Build history of the part. All positions in model axes, mm. A direction names the side the tool comes from. Give positions to 0.01 mm unless a question says otherwise; leave off trailing zeros. Loops run counter-clockwise (first coordinate to the right, second up) from the corner with the lowest first, then second, coordinate; pieces in that order, holes last. Notation, with made-up numbers: (-37, -31.5) -> (4, -31.5) arc R9 ccw to (4, -21.5) -> close; hole circle Ø5 at (68.5, 64.25). An arc over 180 degrees is marked (long way). Answer as a JSON object with one key per item and string values. Group by question number.
Q1. Wall check: probe 1 along X at (y, z) = (-13, 24.5); probe 2 along Y at (x, z) = (7.5, 29.5); probe 3 along Y at (x, z) = (-7, 32). Give the ranges that are in metal, low to high. Write a range as from..to.
Q2. Band-saw the part on B-B, the plane z = 5. Write the cut outline in (x, y), plus the area to 3 significant figures.
Q3. Band-saw the part on D-D, the plane y = -4. Write the cut outline in (x, z).
Q4. Tool access for faces 1 (the flat face through (-25, 0, 18)), 2 (the flat face through (20, 5.75, 31)), 3 (the cylindrical face through (6.026, -11.639, 27.126)): list every direction of +Z, -Z, +X, -X, +Y, -Y with a clear straight run to the whole face (end or side of a thin tool).
Q5. Two-plate mould, pull along Z, no slides. Class faces 4 (the flat face through (20, 5.75, 5)), 5 (the flat face through (8, 13, 18)), 6 (the flat face through (25, 0, 18)): pulls with the +Z half, pulls with the -Z half, needs draft (parallel to the pull), parting line crosses it, or undercut.
Q6. Band-saw the part on A-A, the plane y = 9.5. Write the cut outline in (x, z), plus the area to 3 significant figures.
Q7. Band-saw the part on C-C, the plane x = 7.5. Write the cut outline in (y, z), plus the area to 3 significant figures.
Q8. Drop flat-ended pins along their axis: pin 1 (3 mm diameter, centred on x = -20, z = 31, fed in from +Y); pin 2 (1.2 mm diameter, centred on x = -15.5, y = 1, fed in from +Z); pin 3 (8 mm diameter, centred on x = -6.5, y = 2, fed in from -Z). Give the stop position or say it passes through.
from build123d import *

# Parameters (mm, degrees)
CROQUIS1_W              = 50
CROQUIS1_H              = 31.5
CROQUIS1_R              = 11.25
SALIENTE_EXTRUIR1_DEPTH = 36
CROQUIS2_R              = 1.75
CORTAR_EXTRUIR1_DEPTH   = 10
CROQUIS3_R              = 2
CORTAR_EXTRUIR2_DEPTH   = 18
MATRIZC1_COUNT          = 6


with BuildPart() as part:
    # Croquis1 → Saliente-Extruir1 (new body)
    with BuildSketch(Plane.XY):
        Rectangle(CROQUIS1_W, CROQUIS1_H)
        Circle(CROQUIS1_R, mode=Mode.SUBTRACT)
    extrude(amount=SALIENTE_EXTRUIR1_DEPTH)

    # Croquis2 → Cortar-Extruir1 (cut)
    with BuildSketch(Plane(origin=(0, 15.75, 0), x_dir=(1, 0, 0), z_dir=(0, 1, 0))):
        with Locations(Location((-20, -5, 0), (0, 0, 270))):
            Circle(CROQUIS2_R)
        with Locations(Location((20, -5, 0), (0, 0, 270))):
            Circle(CROQUIS2_R)
        with Locations(Location((20, -31, 0), (0, 0, 270))):
            Circle(CROQUIS2_R)
        with Locations(Location((-20, -31, 0), (0, 0, 270))):
            Circle(CROQUIS2_R)
    extrude(amount=-CORTAR_EXTRUIR1_DEPTH, mode=Mode.SUBTRACT)

    # Croquis3 → Cortar-Extruir2 (cut)
    with BuildSketch(Plane.XY.offset(36)):
        with Locations((-15, 0)):
            Circle(CROQUIS3_R)
    cortar_extruir2 = extrude(amount=-CORTAR_EXTRUIR2_DEPTH, mode=Mode.SUBTRACT)

    # MatrizC1: Cortar-Extruir2 ×6 about axis
    matrizc1_axis = Axis((0, 0, 0), (0, 0, 1))
    for i in range(1, MATRIZC1_COUNT):
        add(cortar_extruir2.rotate(matrizc1_axis, i * 360 / MATRIZC1_COUNT), mode=Mode.SUBTRACT)


solid = part.part
Worked answers:
{
 "1": {"probe 1": "-25..-9.5, -5.5..5.5, 9.5..25", "probe 2": "-15.75..-14.99, -10.99..-8.39, 8.39..10.99, 14.99..15.75", "probe 3": "-15.75..-14.93, -11.05..-8.81, 8.81..11.05, 14.93..15.75"},
 "2": {"outline": "(-25, -15.75) -> (25, -15.75) -> (25, 15.75) -> (21.75, 15.75) -> (21.75, 5.75) -> (18.25, 5.75) -> (18.25, 15.75) -> (-18.25, 15.75) -> (-18.25, 5.75) -> (-21.75, 5.75) -> (-21.75, 15.75) -> (-25, 15.75) -> close; hole circle Ø22.5 at (0, 0)", "area": "1,110 mm2"},
 "3": {"outline": "(-25, 0) -> (-10.51, 0) -> (-10.51, 36) -> (-25, 36) -> close; (10.51, 0) -> (25, 0) -> (25, 36) -> (10.51, 36) -> close"},
 "4": {"face 1": "+Z, -Z, -X, +Y, -Y", "face 2": "+Y", "face 3": "+Z"},
 "5": {"face 4": "undercut", "face 5": "pulls with the +Z half", "face 6": "needs draft"},
 "6": {"outline": "(-25, 0) -> (-6.03, 0) -> (-6.03, 36) -> (-25, 36) -> close; (6.03, 0) -> (25, 0) -> (25, 36) -> (6.03, 36) -> close; hole circle Ø3.5 at (-20, 5); hole circle Ø3.5 at (-20, 31); hole circle Ø3.5 at (20, 5); hole circle Ø3.5 at (20, 31)", "area": "1,330 mm2"},
 "7": {"outline": "(-15.75, 0) -> (-8.39, 0) -> (-8.39, 36) -> (-10.99, 36) -> (-10.99, 18) -> (-14.99, 18) -> (-14.99, 36) -> (-15.75, 36) -> close; (8.39, 0) -> (15.75, 0) -> (15.75, 36) -> (14.99, 36) -> (14.99, 18) -> (10.99, 18) -> (10.99, 36) -> (8.39, 36) -> close", "area": "386 mm2"},
 "8": {"pin 1": "y = 5.75", "pin 2": "z = 18", "pin 3": "through"}
}
